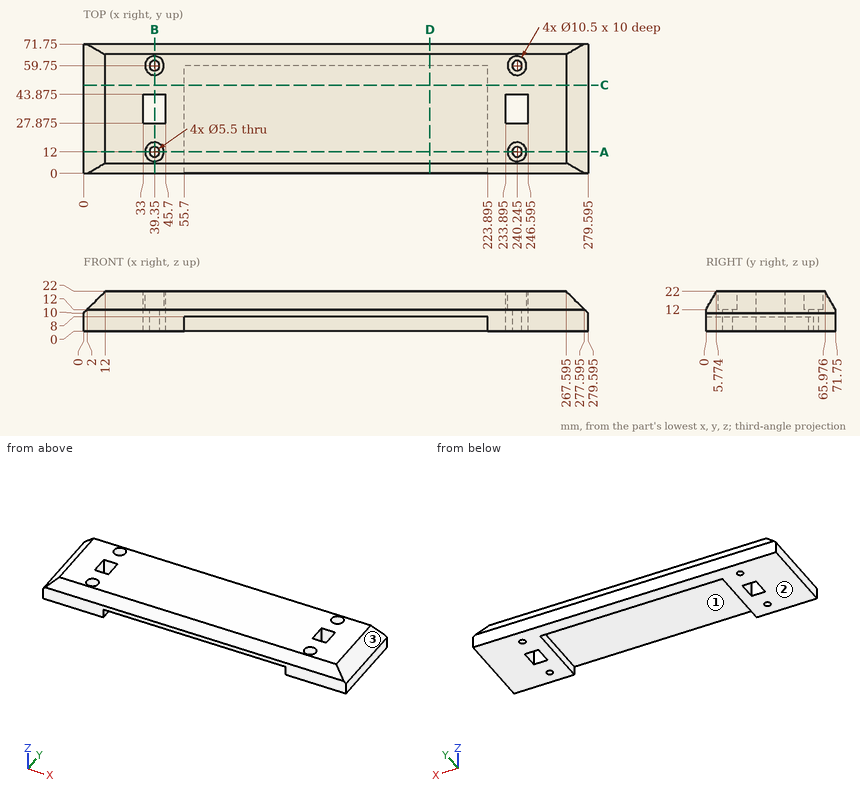
Input: dimensioned drawing with shaded views. Units: mm. Origin: part minimum x, y, z. Round coordinates to 2 decimals unless told otherwise and drop trailing zeros. Order: outer loops, then holes, each group sorted by start corner. A loop starts at its lowest first (then second) coordinate and runs counter-clockwise, first axis right, second up.
Q1. Section B-B, the plane x = 39.35. Give the number of separate pieces and of enclosed holes in the cut face, and give its area (3 significant figures).
Result sheet:
separate pieces: 4
enclosed holes: 0
area: 827 mm2
Q2. Section A-A, the plane y = 12. Output: boundary loops of the cut face in (x, z) (1 decimal), and give its area (3 significant figures).
Result sheet:
outline: (0, 0) - (36.6, 0) - (36.6, 12) - (34.1, 12) - (34.1, 22) - (12, 22) - (0, 10) - close; (42.1, 0) - (55.7, 0) - (55.7, 8) - (223.9, 8) - (223.9, 0) - (237.5, 0) - (237.5, 12) - (235, 12) - (235, 22) - (44.6, 22) - (44.6, 12) - (42.1, 12) - close; (243, 0) - (279.6, 0) - (279.6, 10) - (267.6, 22) - (245.5, 22) - (245.5, 12) - (243, 12) - close
area: 4,320 mm2
Q3. Pin query (flat end, axial travel): pin 1 (10 mm diameter, centred on x = 155.5, z = 18.5, fed in from -Y) (1 decimal); pin 2 (3 mm diameter, centred on x = 121, z = 12.5, fed in from +Y); pin 3 (3 mm diameter, centred on x = 37.5, y = 58, fed in from +Z); pin 4 (4 mm diameter, centred on x = 90, y = 45.5, fed in from -Z). Return the tip coordinate at first contact, or that it passes through.
Result sheet:
pin 1: stops at y = 0.9
pin 2: stops at y = 71.75
pin 3: stops at z = 12
pin 4: stops at z = 8
Q4. Material intervals for probe 1 along X at (y, z) = (34, 3.5) (1 decimal); probe 2 along X at (y, z) = (45.5, 1.25) (1 decimal); probe 3 along X at (y, z) = (29, 15.5) (1 decimal), sorted ascending.
Result sheet:
probe 1: x = 0 to 33, 45.7 to 55.7, 223.9 to 233.9, 246.6 to 279.6
probe 2: x = 0 to 55.7, 223.9 to 279.6
probe 3: x = 5.5 to 33, 45.7 to 233.9, 246.6 to 274.1
Q5. Section D-D, the plane x = 192. Output: boundary loops of the cut face in (y, z).
Result sheet:
outline: (0, 8) - (59.75, 8) - (59.75, 0) - (71.75, 0) - (71.75, 12) - (65.98, 22) - (5.77, 22) - (0, 12) - close
Q6. Mould query, pull axis X, two halves, no side actions, for the marked faces 1, 2 and 3. Classes: released by +X, released by -X, zero draft, split by the parting line, or undercut.
Result sheet:
face 1: undercut
face 2: zero draft
face 3: released by +X
Q7. Section C-C, the plane y = 49. Output: boundary loops of the cut face in (x, z) (1 decimal).
Result sheet:
outline: (0, 0) - (55.7, 0) - (55.7, 8) - (223.9, 8) - (223.9, 0) - (279.6, 0) - (279.6, 10) - (267.6, 22) - (12, 22) - (0, 10) - close
